Read the model definition and answer for the solid it produces. Units are mm, in the model's axes. Give positions to 0.01 mm unless a question says otherwise; leave off trailing zeros. Loops run counter-clockwise (first coordinate to the right, second up) from the corner with the lowest first, then second, coordinate; pieces in that order, holes last.
(1) Find section C-C, the plane z = 14. Write down the section's boundary in (x, y), then the cut area to 3 significant figures.
(2) Find section B-B, the plane y = 0.6. Write down the section's boundary in (x, z).
(3) Straight lines are drawn through the part: probe 1 along Z at (x, y) = (0.65, -0.4); probe 2 along Y at (x, z) = (-0.4, 6.5); probe 3 along Y at (x, z) = (0.1, 9.5). For each, find the intervals that lie inside material, in ascending order.
(4) Find section A-A, the plane x = 0. Write down the section's boundary in (y, z).
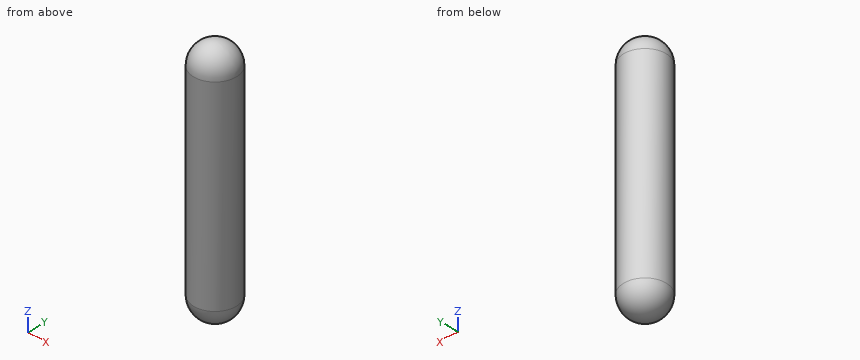
Autodesk Inventor part; units mm, degrees
ref_plane "YZ Plane" through (0, 0, 0) normal (1, 0, 0) x (0, 1, 0)
ref_plane "XZ Plane" through (0, 0, 0) normal (0, 1, 0) x (-1, 0, 0)
ref_plane "XY Plane" through (0, 0, 0) normal (0, 0, 1) x (1, 0, 0)
sketch "Sketch1" plane through (0, 0, 0) normal (0, 0, 1) x (1, 0, 0)
  circle A0 centre (0, 0) radius 2
  dimension "d0" = 4
extrude "Extrusion1" add sketch "Sketch1" along normal blind 23
fillet "Fillet1" radius 2 2 edges at (-2, 0, 23) (-2, 0, 0)
scale "Scale1" factors (0.5, 0.5, 0.5) then translate (0, 0, 5.75) bodies 1
properties part number "Pasador 2"
Entries:
1. outline: circle Ø2 at (0, 0)
1. area: 3.14 mm2
2. outline: (-0.8, 6.75) arc R0.8 ccw to (0.8, 6.75) - (0.8, 16.25) arc R0.8 ccw to (-0.8, 16.25) - close
3. probe 1: z = 6.1 to 16.9
3. probe 2: y = -0.88 to 0.88
3. probe 3: y = -0.99 to 0.99
4. outline: (-1, 6.75) arc R1 ccw to (1, 6.75) - (1, 16.25) arc R1 ccw to (-1, 16.25) - close
